Autodesk Inventor part; units mm, degrees
ref_plane "MSC_PF1" through (0, 0, 0) normal (1, 0, 0) x (0, 1, 0)
ref_plane "MSC_PT1" through (3.9, 0, -0.58) normal (0, 0, -1) x (-1, 0, 0)
ref_plane "YZ Plane" through (0, 0, 0) normal (1, 0, 0) x (0, 1, 0)
sketch "Sketch2" plane through (0, 0, 0) normal (0, 1, 0) x (-1, 0, 0)
  line L0 (0, -14) -> (-2, -14)
  line L1 (0, 0) -> (0, -14)
  line L2 (-3.9, 0) -> (0, 0)
  line L3 (-3.9, -0.58) -> (-3.9, 0)
  line L4 (-2, -2.48) -> (-3.9, -0.58)
  line L5 (-2, -14) -> (-2, -2.48)
  line L6 (0, 0) -> (0, -14)
  dimension "d2" = 45
  dimension "d4" = 2
  dimension "d6" = 3.9
  dimension "d8" = 2.48
  dimension "d10" = 14
revolve "Revolution1" add sketch "Sketch2" angle 360 about axis through (0, 0, 0) along (0, 0, -1)
fillet "Fillet1" radius 0.35 1 edges at (-2, 0, -2.48)
chamfer "Chamfer1" distance 0.35 angle 45 1 edges at (-2, 0, -14)
sketch "Sketch4" plane through (0, 0, 0) normal (0, 0, 1) x (1, 0, 0)
  circle A0 centre (0, 0) radius 3.9
  circle A1 centre (0, 0) radius 1.25 construction
  line L0 (-1.25, -0.7217) -> (-1.25, 0.7217)
  line L1 (-1.25, 0.7217) -> (0, 1.4434)
  line L2 (0, 1.4434) -> (1.25, 0.7217)
  line L3 (1.25, 0.7217) -> (1.25, -0.7217)
  line L4 (1.25, -0.7217) -> (0, -1.4434)
  line L5 (0, -1.4434) -> (-1.25, -0.7217)
  dimension "d27" = 2.5
extrude "Extrusion1" cut sketch "Sketch4" against normal blind 1.5 contours L0 L1 L2 L3 L4 L5
sketch "Sketch5" plane through (0, 0, 0) normal (0, 0, 1) x (1, 0, 0)
  circle A0 centre (0, 0) radius 3.9
  circle A1 centre (0, 0) radius 1.2625
  dimension "d38" = 2.525
extrude "Extrusion2" cut sketch "Sketch5" against normal blind 1.5 contours A1
thread "Thread1"
ref_plane "MSC_PF1" through (0, 0, 0) normal (1, 0, 0) x (0, 1, 0)
ref_plane "MSC_PT1" through (3.9, 0, -0.58) normal (0, 0, -1) x (-1, 0, 0)
equation "\"d24\" = Rr"
equation "\"d25\" = 0.5 * PTC"
equation "\"d26\" = 0.5 * PTC"
equation "\"d38\" = 1.01 * ParJ"
equation "\"d39\" = Tt"
equation "\"d4\" = 0.5 * NND"
equation "\"d6\" = 0.5 * ParA"
equation "\"d8\" = ParH"
equation "\"d10\" = NLG"
equation "\"d27\" = ParJ"
equation "\"d28\" = Tt"
equation "\"d31\" = Lt"
equation "\"NND\" = 4"
equation "\"NLG\" = 14"
equation "\"PTC\" = 0.7"
equation "\"ParA\" = 7.8"
equation "\"ParH\" = 2.48"
equation "\"ParJ\" = 2.5"
equation "\"Tt\" = 1.5"
equation "\"Rr\" = 0.35"
equation "\"msp_e\" = 0.288675 * ParJ"
equation "\"Lt\" = 10.12"
equation "\"THREADDIA\" = NND"
properties part number "ASME/ANSI B18.3.5M - M4x14(2)" material "Steel, Mild"
Verification items for the finished model (mm, model axes). A direction names the side the tool comes from. Give positions to 0.01 mm unless a question says otherwise; leave off trailing zeros. Order: outer loops, then holes, each group sorted by start corner. A loop starts at its lowest first (then second) coordinate and runs counter-clockwise, first axis right, second up. Notation, with made-up numbers: (1.5, -28.5) -> (33.5, -28.5) arc R13 ccw to (33.5, -24.5) -> close; hole circle Ø1 at (64.25, 52.25). An arc over 180 degrees is marked (long way). Answer as CSV lines item,"result".
Q1. Sectioned sample at B-B on z = -6.75. Record the cut outline in (x, y).
Solutions:
outline,"circle Ø4 at (0, 0)"
Q2. Scan lines: probe 1 along Z at (x, y) = (0.5, -0.5); probe 2 along X at (y, z) = (1.25, -10.75); probe 3 along Y at (x, z) = (0.75, -8.25). Record each from-to range of solid material in increasing order.
Solutions:
probe 1,"z = -14 to -1.5"
probe 2,"x = -1.56 to 1.56"
probe 3,"y = -1.85 to 1.85"
Q3. Access from +Z, -Z, +X, -X, +Y, -Y to the whole of each face (thin tool, end or side, straight path). Record for faces 4 (the flat face through (2, 0, 0)), 5 (the cylindrical face through (0, -2, -8)).
Solutions:
face 4,"+Z, +X, -X, +Y, -Y"
face 5,"-Z"
Q4. Release check for a two-part mould opening along X. For faces 1 (the conical face through (-0.48, -2.16, -2.27)), 2 (the flat face through (0, 0, -14)), 3 (the flat face through (0, 0, -1.5)) record: +X half, -X half, draft (parallel to the pull), parting line (faces both ways), or undercut.
Solutions:
face 1,"parting line"
face 2,"draft"
face 3,"undercut"
Q5. Depth check by flat-ended pin: pin 1 (1.5 mm diameter, centred on x = -3, y = 1, fed in from -Z); pin 2 (1.3 mm diameter, centred on x = -0.5, y = 0, fed in from +Z); pin 3 (1.5 mm diameter, centred on x = 1.5, z = -11.5, fed in from -Y). Enter the tip coordinate at first touch or a pass-through.
Solutions:
pin 1,"stops at z = -2.07"
pin 2,"stops at z = -1.5"
pin 3,"stops at y = -1.85"
